from build123d import *

# Parameters (mm, degrees)
SKETCH1_W                                  = 100
SKETCH1_H                                  = 170
BODY_DEPTH                                 = 3
REDUCESOMEWIDTH_DEPTH                      = 7
SCREWHEADHOLECARRIAGEY_R                   = 5
CUTFOROTHERSCREWSHEADS_DEPTH               = 7
ENDMILLMINIMUMRADIUS_R                     = 3.5
F_3_5_3_5_CABLETIEHOLES_D                  = 3.5
F_4_2_4_2_KP8_HOLES1_D                     = 4.2
F_4_2_4_2_KP8_HOLES2_D                     = 4.2
F_5_2_5_2_MOUNTANGLECORNERHOLES_AT_2_COUNT = 2
F_5_2_5_2_MOUNTANGLECORNERHOLES_AT_2_PITCH = 20
F_5_2_5_2_MOUNTANGLECORNERHOLES_AT_3_COUNT = 2
F_5_2_5_2_MOUNTANGLECORNERHOLES_AT_3_PITCH = 80
F_5_2_5_2_MOUNTANGLECORNERHOLES_AT_4_COUNT = 2
F_5_2_5_2_MOUNTANGLECORNERHOLES_AT_4_PITCH = 82.462112512
F_5_2_5_2_SK8_MOUNT_HOLES_D                = 5.2
F_5_2_5_2_SK8_MOUNT_HOLES_CSINK_D          = 11.5
F_5_2_5_2_SK8_MOUNT_HOLES_CSINK_ANGLE      = 90
F_3_5_3_5_ENDSENSORSHOLES_D                = 3.5
F_3_5_3_5_ENDSENSORSHOLES_CSINK_D          = 6.5
F_3_5_3_5_ENDSENSORSHOLES_CSINK_ANGLE      = 90
F_5_2_5_2_MOUNTTOBASEHOLES_D               = 5.2


with BuildPart() as part:
    # Sketch1 → Body (new body, symmetric)
    with BuildSketch(Plane.XY):
        Polygon((50, 0), (-50, 0), (-35.5, -14.5), (35.5, -14.5), align=None)
        with Locations((0, 85)):
            Rectangle(SKETCH1_W, SKETCH1_H)
    extrude(amount=BODY_DEPTH, both=True)

    # Sketch6 → ReduceSomeWidth (cut, through all)
    with BuildSketch(Plane.XY.offset(3)):
        Polygon((-50, 115), (-47, 112), (-47, 17), (-50, 14), align=None)
        Polygon((50, 115), (47, 112), (47, 17), (50, 14), align=None)
    extrude(amount=-REDUCESOMEWIDTH_DEPTH, mode=Mode.SUBTRACT)

    # screwHeadHoleCarriageY → CutForOtherScrewsHeads (cut, through all)
    with BuildSketch(Plane(origin=(0, 0, -3), x_dir=(-1, 0, 0), z_dir=(0, 0, -1))):
        with Locations((-27, 12)):
            Circle(SCREWHEADHOLECARRIAGEY_R)
        with Locations((27, 12)):
            Circle(SCREWHEADHOLECARRIAGEY_R)
        with BuildLine():
            Line((-32, 70.2), (-32, 72.7))
            ThreePointArc((-32, 72.7), (-27, 77.7), (-22, 72.7))
            Line((-22, 72.7), (-22, 70.2))
            ThreePointArc((-22, 70.2), (-27, 65.2), (-32, 70.2))
        make_face()
        with BuildLine():
            Line((22, 70.2), (22, 72.7))
            ThreePointArc((22, 72.7), (27, 77.7), (32, 72.7))
            Line((32, 72.7), (32, 70.2))
            ThreePointArc((32, 70.2), (27, 65.2), (22, 70.2))
        make_face()
    extrude(amount=-CUTFOROTHERSCREWSHEADS_DEPTH, mode=Mode.SUBTRACT)

    # EndMillMinimumRadius
    endmillminimumradius_edges = [part.edges().sort_by_distance(p)[0] for p in [
        (50, 170, 0),
        (50, 0, 0),
        (35.5, -14.5, 0),
        (-35.5, -14.5, 0),
        (-50, 0, 0),
        (-50, 170, 0),
        (-50, 14, 0),
        (-50, 115, 0),
        (-47, 112, 0),
        (-47, 17, 0),
        (50, 115, 0),
        (50, 14, 0),
        (47, 17, 0),
        (47, 112, 0),
    ]]
    fillet(endmillminimumradius_edges, radius=ENDMILLMINIMUMRADIUS_R)

    # Ø3.5 (3.5) CableTieHoles (through all)
    with Locations(Plane(origin=(0, 0, -3), x_dir=(-1, 0, 0), z_dir=(0, 0, -1))):
        with Locations((-45.5, 122), (45.5, 122)):
            Hole(F_3_5_3_5_CABLETIEHOLES_D / 2)

    # Ø4.2 (4.2) KP8 Holes1 (through all)
    with Locations(Plane(origin=(0, 0, -3), x_dir=(-1, 0, 0), z_dir=(0, 0, -1))):
        with Locations((-21, 159), (21, 159)):
            Hole(F_4_2_4_2_KP8_HOLES1_D / 2)

    # Ø4.2 (4.2) KP8 Holes2 (through all)
    with Locations(Plane(origin=(0, 0, -3), x_dir=(-1, 0, 0), z_dir=(0, 0, -1))):
        with Locations((-21, -8), (21, -8)):
            Hole(F_4_2_4_2_KP8_HOLES2_D / 2)

    # Sketch16 → Ø5.2 (5.2) MountAngleCornerHoles (revolve, cut)
    with BuildSketch(Plane(origin=(40, 154, -3), x_dir=(0, 1, 0), z_dir=(1, 0, 0))):
        Polygon((0, 0), (0, 6), (5.75, 6), (2.6, 2.85), (2.6, 0), align=None)
    f_5_2_5_2_mountanglecornerholes = revolve(axis=Axis((40, 154, -9.35), (0, 0, 1)), mode=Mode.SUBTRACT)

    # Ø5.2 (5.2) MountAngleCornerHoles at 2: Ø5.2 (5.2) MountAngleCornerHoles ×2
    with Locations(*[(0, -i * F_5_2_5_2_MOUNTANGLECORNERHOLES_AT_2_PITCH, 0) for i in range(1, F_5_2_5_2_MOUNTANGLECORNERHOLES_AT_2_COUNT)]):
        add(f_5_2_5_2_mountanglecornerholes, mode=Mode.SUBTRACT)

    # Ø5.2 (5.2) MountAngleCornerHoles at 3: Ø5.2 (5.2) MountAngleCornerHoles ×2
    with Locations(*[(-i * F_5_2_5_2_MOUNTANGLECORNERHOLES_AT_3_PITCH, 0, 0) for i in range(1, F_5_2_5_2_MOUNTANGLECORNERHOLES_AT_3_COUNT)]):
        add(f_5_2_5_2_mountanglecornerholes, mode=Mode.SUBTRACT)

    # Ø5.2 (5.2) MountAngleCornerHoles at 4: Ø5.2 (5.2) MountAngleCornerHoles ×2
    with Locations(*[Vector(-0.9701425, -0.242535625, 0) * (i * F_5_2_5_2_MOUNTANGLECORNERHOLES_AT_4_PITCH) for i in range(1, F_5_2_5_2_MOUNTANGLECORNERHOLES_AT_4_COUNT)]):
        add(f_5_2_5_2_mountanglecornerholes, mode=Mode.SUBTRACT)

    # Ø5.2 (5.2) SK8 Mount Holes (through all)
    with Locations(Plane(origin=(0, 0, -3), x_dir=(-1, 0, 0), z_dir=(0, 0, -1))):
        with Locations((-45, 143.1), (-13, 143.1), (13, 143.1), (45, 143.1), (-45, 7), (-13, 7), (13, 7), (45, 7)):
            CounterSinkHole(F_5_2_5_2_SK8_MOUNT_HOLES_D / 2, F_5_2_5_2_SK8_MOUNT_HOLES_CSINK_D / 2, counter_sink_angle=F_5_2_5_2_SK8_MOUNT_HOLES_CSINK_ANGLE)

    # Ø3.5 (3.5) EndSensorsHoles (through all)
    with Locations(Plane(origin=(0, 0, -3), x_dir=(-1, 0, 0), z_dir=(0, 0, -1))):
        with Locations((-43, 49.5), (-36, 49.5), (36, 98.5), (43, 98.5)):
            CounterSinkHole(F_3_5_3_5_ENDSENSORSHOLES_D / 2, F_3_5_3_5_ENDSENSORSHOLES_CSINK_D / 2, counter_sink_angle=F_3_5_3_5_ENDSENSORSHOLES_CSINK_ANGLE)

    # Ø5.2 (5.2) MountToBaseHoles (through all)
    with Locations(Plane.XY.offset(3)):
        with Locations((-38.3, 110.2), (-38.3, 65.2), (-38.3, 20.2), (38.3, 20.2), (38.3, 65.2), (38.3, 110.2)):
            Hole(F_5_2_5_2_MOUNTTOBASEHOLES_D / 2)


solid = part.part
The model under review builds one solid part; all positions refer to its coordinate system, in mm. A direction names the side the tool comes from. Give positions to 0.01 mm unless a question says otherwise; leave off trailing zeros. Order: outer loops, then holes, each group sorted by start corner. A loop starts at its lowest first (then second) coordinate and runs counter-clockwise, first axis right, second up. Notation, with made-up numbers: M -3,-21 L 24,-21 A23 ccw 24,-1 Z; hole C 79.25,76.5 d6. An arc over 180 degrees is marked long. One line per question, with ' | ' between items. Start each with the question number.
1) Mouldability with a two-part tool opening along Y and no side actions: class faces 3 (the face through (-40.12, 151.25, 0)), 4 (the face through (-26.9, 77.7, 0)), 5 (the face through (48.95, 169, -0.04)), 6 (the face through (0, -14.5, 0)) as pulls with the +Y half, pulls with the -Y half, needs draft (parallel to the pull), parting line crosses it, or undercut.
2) Consider section D-D, the plane y = 104. Give the boundary of the cut face in (x, z), then the cut area to 3 significant figures.
3) Consider section C-C, the plane y = 143.1. Give the boundary of the cut face in (x, z).
4) Wall thickness on L1, parallel to Y at x = -21, z = 1.5; L2, parallel to X at y = 154, z = -1.15; L3, parallel to Y at x = 27, z = -0.5: over which ranges is each line inside the solid? List them lowest first. Write a range as from..to.
5) Clearance check with flat-ended pins moving along their axes: P1, Ø5, axis at x = 21, y = -8, coming from the -Z side; P2, Ø6, axis at x = -40, y = 134, coming from the +Z side; P3, Ø3, axis at y = 71, z = -1, coming from the -X side. State where each tip first meets the part, or that it passes through.
6) Consider section A-A, the plane x = -13. Give the boundary of the cut face in (y, z).
7) Consider section B-B, the plane y = -8. Give the boundary of the cut face in (x, z), then the cut area to 3 significant figures.
8) For faces 1 (the face through (-27.1, 65.2, 0)), 2 (the face through (-42.46, 142.05, 0)), list the 3-axis set-ups (+Z, -Z, +X, -X, +Y, -Y) from which the entire face can be reached by the end or side of a thin tool; tool diameter is ignored.
Found:
1) face 3: undercut | face 4: undercut | face 5: pulls with the +Y half | face 6: pulls with the -Y half
2) outline: M -47,-3 L 47,-3 L 47,3 L -47,3 Z | area: 564 mm²
3) outline: M -50,-2.25 L -47.6,0.15 L -47.6,3 L -50,3 Z; M -42.4,0.15 L -39.25,-3 L -18.75,-3 L -15.6,0.15 L -15.6,3 L -42.4,3 Z; M -10.4,0.15 L -7.25,-3 L 7.25,-3 L 10.4,0.15 L 10.4,3 L -10.4,3 Z; M 15.6,0.15 L 18.75,-3 L 39.25,-3 L 42.4,0.15 L 42.4,3 L 15.6,3 Z; M 47.6,0.15 L 50,-2.25 L 50,3 L 47.6,3 Z
4) L1: y = -14.5..-10.1, -5.9..156.9, 161.1..170 | L2: x = -50..-42.6, -37.4..37.4, 42.6..50 | L3: y = -14.5..7, 17..65.2, 77.7..170
5) P1: stops at z = -3 | P2: stops at z = 0.25 | P3: stops at x = -47
6) outline: M -14.5,-3 L 1.25,-3 L 4.4,0.15 L 4.4,3 L -14.5,3 Z; M 9.6,0.15 L 12.75,-3 L 137.35,-3 L 140.5,0.15 L 140.5,3 L 9.6,3 Z; M 145.7,0.15 L 148.85,-3 L 170,-3 L 170,3 L 145.7,3 Z
7) outline: M -42,-3 L -23.1,-3 L -23.1,3 L -42,3 Z; M -18.9,-3 L 18.9,-3 L 18.9,3 L -18.9,3 Z; M 23.1,-3 L 42,-3 L 42,3 L 23.1,3 Z | area: 454 mm²
8) face 1: +Z, -Z | face 2: -Z
